The listing builds one solid part. Answer for the finished solid, in the listing's coordinates (mm). A direction names the side the tool comes from. Round coordinates to 2 decimals unless told otherwise and drop trailing zeros. Write each loop counter-clockwise with the first axis right and the second up, starting at its lowest first coordinate (ties: lowest second). Pieces come first, ordered by that corner, then holes.
Item 1: A tool of negligible diameter and unlimited length cuts with its end or side. For faces 5 (the face through (19, 2, 0)), 6 (the face through (-23, 2, 0)), 7 (the face through (21, 2, -23)), 8 (the face through (-23, 2, -15.5)), from which of +Z, -Z, +X, -X, +Y, -Y can it reach the whole face along a straight path? Write none if from no direction.
Item 2: Find section B-B on z = 1. Give the vertices of the cut face in (x, y), then the cut area to 3 significant figures.
Item 3: Each of these flat-tipped pins is pushed along its axis until it touches: pin 1 (2 mm diameter, centred on y = 2.5, z = -19.5, fed in from -X); pin 2 (2 mm diameter, centred on y = 2, z = -6, fed in from +X); pin 3 (2 mm diameter, centred on x = -23.5, y = 2, fed in from -Z). Where does it stop, or does it pass through?
Item 4: Find section A-A on y = 1.25. Give the vertices of the cut face in (x, z).
Item 5: For a pull along Z with two mould halves and no side action, classify faces 1 (the face through (0, 2, -31)), 2 (the face through (0, 2, 15.5)), 3 (the face through (-25.5, 2, -8)), 4 (the face through (19, 2, -15.5)) as +Z half, -Z half, draft (parallel to the pull), parting line (faces both ways), or undercut.
Item 6: Find the intervals of material crossed by probe 1 along X at (y, z) = (0.35, -24.5); probe 2 along X at (y, z) = (4.2, -5); probe 3 along Z at (x, y) = (-22, 3.8), in increasing order.
```python
from build123d import *

# Parameters (mm, degrees)
BOSS_EXTRUDE1_DEPTH = 4.5
SKETCH2_W           = 51.255573275
SKETCH2_H           = 30.547230998
CUT_EXTRUDE1_DEPTH  = 5.5


with BuildPart() as part:
    # Sketch1 → Boss-Extrude1 (new body)
    with BuildSketch(Plane(origin=(0, 0, 0), x_dir=(1, 0, 0), z_dir=(0, 1, 0))):
        Polygon((-21, 0), (-21, -15.5), (-25.5, -15.5), (-25.5, -31), (-21, -31), (-21, -35.5), (-16.5, -35.5), (-16.5, -31), (0, -31), (0, -35.5), (4.5, -35.5), (4.5, -31), (16.5, -31), (16.5, -15.5), (21, -15.5), (21, 0), (16.5, 0), (16.5, 15.5), (21, 15.5), (21, 31), (-21, 31), (-21, 15.5), (-25.5, 15.5), (-25.5, 0), align=None)
    extrude(amount=BOSS_EXTRUDE1_DEPTH)

    # Sketch2 → Cut-Extrude1 (cut, through all)
    with BuildSketch(Plane(origin=(0, 4.5, 0), x_dir=(1, 0, 0), z_dir=(0, 1, 0))):
        with Locations((0.127786638, -30.773615499)):
            Rectangle(SKETCH2_W, SKETCH2_H)
    extrude(amount=-CUT_EXTRUDE1_DEPTH, mode=Mode.SUBTRACT)


solid = part.part
```
Check values:
1. face 5: +X, +Y, -Y
1. face 6: +Z, -X, +Y, -Y
1. face 7: +Z, -Z, +X, +Y, -Y
1. face 8: -Z, -X, +Y, -Y
2. outline: (-21, 0) - (21, 0) - (21, 4.5) - (-21, 4.5) - close
2. area: 189 mm2
3. pin 1: stops at x = -21
3. pin 2: stops at x = 16.5
3. pin 3: stops at z = -15.5
4. outline: (-25.5, -15.5) - (-21, -15.5) - (-21, -31) - (21, -31) - (21, -15.5) - (16.5, -15.5) - (16.5, 0) - (21, 0) - (21, 15.5) - (-21, 15.5) - (-21, 0) - (-25.5, 0) - close
5. face 1: -Z half
5. face 2: +Z half
5. face 3: draft
5. face 4: undercut
6. probe 1: x = -21 to 21
6. probe 2: x = -25.5 to 16.5
6. probe 3: z = -15.5 to 0
